Geometry: see drawing. Coordinates: mm, zero at the bounding-box minimum. A direction names the side the tool comes from. Coordinates: 2 decimals unless noted, no trailing zeros. Order: outer loops, then holes, each group sorted by start corner. A loop starts at its lowest first (then second) coordinate and runs counter-clockwise, first axis right, second up.
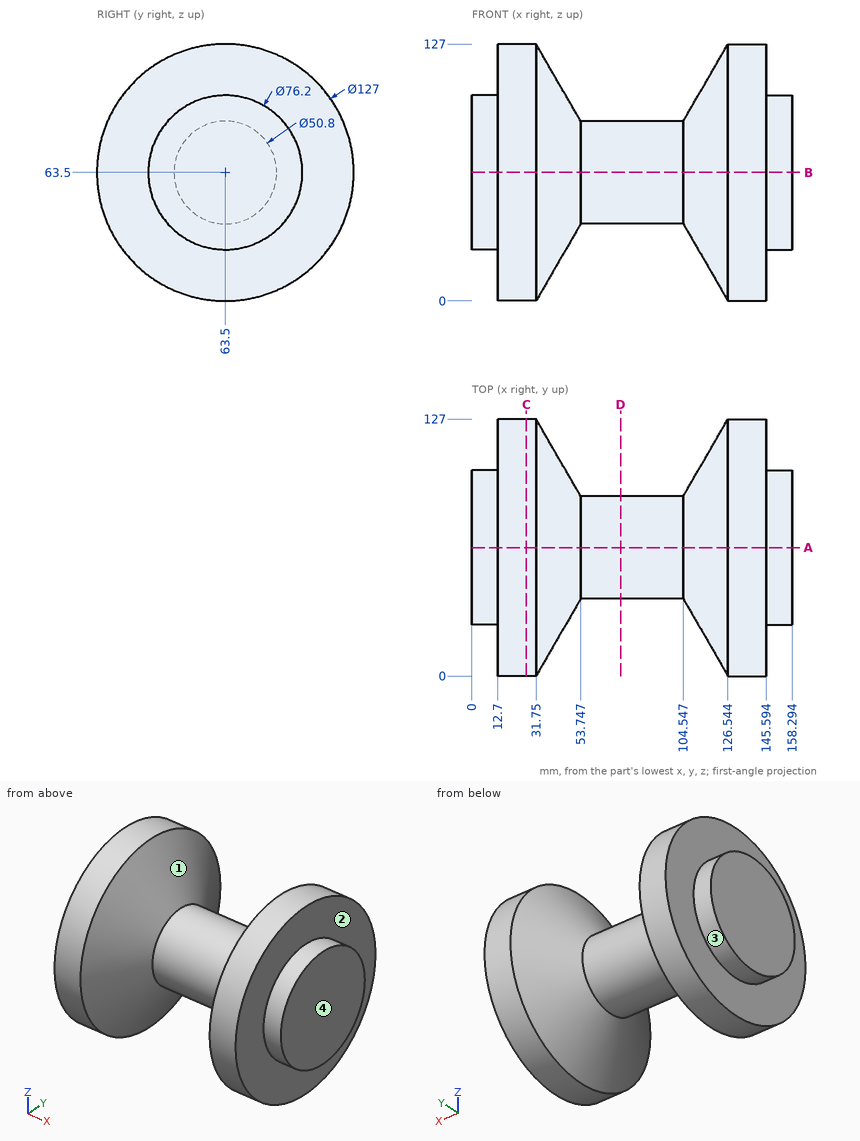
Q1. Section query A-A on y = 63.5. Output: boundary loops of the cut face in (x, z), plus the area to 3 significant figures.
Solutions:
outline: (0, 25.4) - (12.7, 25.4) - (12.7, 0) - (31.75, 0) - (53.75, 38.1) - (104.55, 38.1) - (126.54, 0) - (145.59, 0) - (145.59, 25.4) - (158.29, 25.4) - (158.29, 101.6) - (145.59, 101.6) - (145.59, 127) - (126.54, 127) - (104.55, 88.9) - (53.75, 88.9) - (31.75, 127) - (12.7, 127) - (12.7, 101.6) - (0, 101.6) - close
area: 13,300 mm2
Q2. Set-up query: the marked faces 1, 2, 3 and 4. Return all of +Z, -Z, +X, -X, +Y, -Y with unobstructed straight access to the full face (end or side cutting, diameter ignored); none if empty.
Solutions:
face 1: none
face 2: +X
face 3: -X
face 4: +Z, -Z, +X, +Y, -Y
Q3. Section query D-D on x = 73.5. Output: boundary loops of the cut face in (y, z).
Solutions:
outline: circle Ø50.8 at (63.5, 63.5)
Q4. Material intervals for line 1 along X through (y, z) = (105, 65); line 2 along X through (y, z) = (25.5, 74); line 3 along Y through (x, z) = (37, 83), sorted ascending.
Solutions:
line 1: x = 12.7 to 44.44, 113.86 to 145.59
line 2: x = 12.7 to 45.65, 112.64 to 145.59
line 3: y = 12.71 to 114.29
Q5. Pin query (flat end, axial travel): P1, Ø3, axis at x = 120, y = 31, coming from the -Z side; P2, Ø1.5, axis at x = 83.5, y = 91.5, coming from the +Z side; P3, Ø12, axis at x = 27.5, y = 112.5, coming from the +Z side; P4, Ø8, axis at x = 73.5, y = 42, coming from the +Z side. Return the tip coordinate at first contact, or that it passes through.
Solutions:
P1: stops at z = 19.24
P2: passes through
P3: stops at z = 110.23
P4: stops at z = 81.91
Q6. Section query C-C on x = 27. Output: boundary loops of the cut face in (y, z), plus the area to 3 significant figures.
Solutions:
outline: circle Ø127 at (63.5, 63.5)
area: 12,700 mm2
